Geometry: see drawing. Coordinates: mm, zero at the bounding-box minimum. A direction names the side the tool comes from. Coordinates: 2 decimals unless noted, no trailing zeros. Order: outer loops, then holes, each group sorted by start corner. A loop starts at its lowest first (then second) coordinate and runs counter-clockwise, first axis right, second up.
Item 1: Reachability of the marked faces 3 and 4 from +Z, -Z, +X, -X, +Y, -Y: full face, straight path, thin tool, end or side. Return the list, or none.
Item 2: Ray query, line 1 (Z direction, x = 7.75, y = 7) (3 decimals); line 2 (Z direction, x = 20.5, y = 8.5). Return the intervals inside material, ascending.
Item 3: Section A-A on z = 7. Return the cut outline in (x, y) (3 decimals).
Item 4: Mould query, pull axis Z, two halves, no side actions, for the marked faces 1 and 2. Classes: released by +Z, released by -Z, zero draft, split by the parting line, or undercut.
Item 5: Section C-C on x = 18. Return the cut outline in (y, z) (3 decimals), then the cut area to 3 significant figures.
Item 6: Section B-B on x = 3. Return the cut outline in (y, z) (3 decimals).
Item 7: Contact query for flat-ended pins moving along their axis: P1, Ø3, axis at x = 13, y = 10, coming from the +Z side; P2, Ø6, axis at x = 16.5, z = 2.5, coming from the +Y side; P3, Ø1, axis at x = 7.5, z = 2.5, coming from the +Y side. Output: stop coordinate, or through.
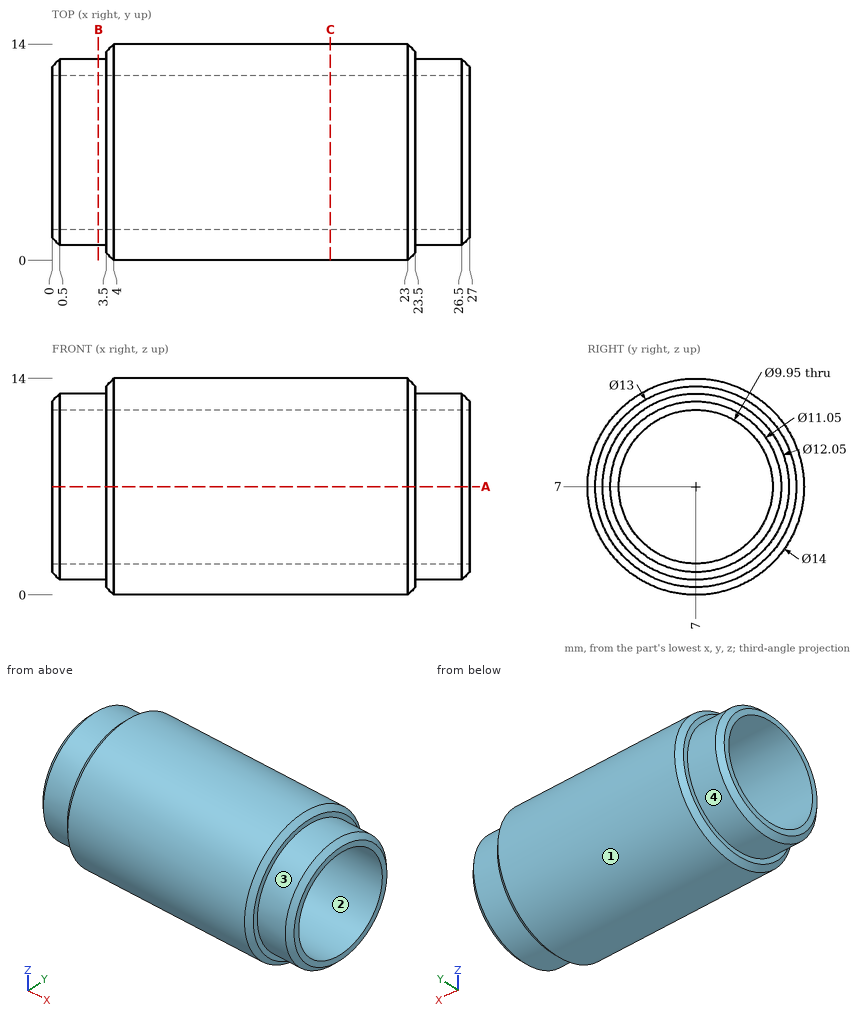
Answer list:
1. face 3: +X
1. face 4: -X
2. line 1: z = 0 to 2.025, 11.975 to 14
2. line 2: z = 0.16 to 2.26, 11.74 to 13.84
3. outline: (0, 1.475) - (0.5, 0.975) - (3.5, 0.975) - (3.5, 0.5) - (4, 0) - (23, 0) - (23.5, 0.5) - (23.5, 0.975) - (26.5, 0.975) - (27, 1.475) - (27, 2.025) - (0, 2.025) - close; (0, 11.975) - (27, 11.975) - (27, 12.525) - (26.5, 13.025) - (23.5, 13.025) - (23.5, 13.5) - (23, 14) - (4, 14) - (3.5, 13.5) - (3.5, 13.025) - (0.5, 13.025) - (0, 12.525) - close
4. face 1: split by the parting line
4. face 2: undercut
5. outline: circle Ø14 at (7, 7); hole circle Ø9.95 at (7, 7)
5. area: 76.2 mm2
6. outline: circle Ø12.05 at (7, 7); hole circle Ø9.95 at (7, 7)
7. P1: stops at z = 13.84
7. P2: stops at y = 13.84
7. P3: stops at y = 12.74
